Verification items for the finished model (mm, model axes). A direction names the side the tool comes from. Give positions to 0.01 mm unless a question says otherwise; leave off trailing zeros.
from build123d import *

# Parameters (mm, degrees)
SKETCH3_R         = 2.54
CAMERA_LENS_DEPTH = 2.54
SKETCH4_W         = 15.24
SKETCH4_H         = 10.16
CAMERA_BODY_DEPTH = 6.35


with BuildPart() as part:
    # Sketch2 → FOV section 0
    with BuildSketch(Plane(origin=(0, 90.932, 0), x_dir=(1, 0, 0), z_dir=(0, 1, 0))):
        with BuildLine():
            Line((-2.755394972, -1.722121857), (2.755394972, -1.722121857))
            Line((2.755394972, -1.722121857), (2.755394972, 1.722121857))
            Line((2.755394972, 1.722121857), (-2.755394972, 1.722121857))
            Line((-2.755394972, 1.722121857), (-2.755394972, -1.722121857))
        make_face()
    # Sketch1 → FOV section 1
    with BuildSketch(Plane(origin=(0, 0, 0), x_dir=(1, 0, 0), z_dir=(0, 1, 0))):
        with BuildLine():
            Line((-101.6, -63.5), (101.6, -63.5))
            Line((101.6, -63.5), (101.6, 63.5))
            Line((101.6, 63.5), (-101.6, 63.5))
            Line((-101.6, 63.5), (-101.6, -63.5))
        make_face()
    loft()

    # Sketch3 → camera lens (add)
    with BuildSketch(Plane(origin=(0, 90.932, 0), x_dir=(1, 0, 0), z_dir=(0, 1, 0))):
        with Locations(Location((0, 0, 0), (0, 0, 137.312390012))):
            Circle(SKETCH3_R)
    extrude(amount=CAMERA_LENS_DEPTH)

    # Sketch4 → camera body (add)
    with BuildSketch(Plane(origin=(0, 93.472, 0), x_dir=(1, 0, 0), z_dir=(0, 1, 0))):
        Rectangle(SKETCH4_W, SKETCH4_H)
    extrude(amount=CAMERA_BODY_DEPTH)


solid = part.part
(1) Release check for a two-part mould opening along Y. For faces 1 (the flat face through (0, 99.822, 0)), 2 (the cylindrical face through (-2.3, 92.18, -1.08)), 3 (the flat face through (7.62, 97, 0)) record: pulls with the +Y half, pulls with the -Y half, needs draft (parallel to the pull), parting line crosses it, or undercut.
Solved:
face 1: pulls with the +Y half
face 2: undercut
face 3: needs draft
(2) Set-up check for faces 4 (the flat face through (-7.62, 97, 0)), 5 (the flat face through (0, 97, -5.08)), 6 (the flat face through (0, 97, 5.08)): record each of +Z, -Z, +X, -X, +Y, -Y from which the full face is reachable in a straight line by a thin tool's end or side.
Solved:
face 4: +Z, -Z, -X, +Y
face 5: -Z, +X, -X, +Y
face 6: +Z, +X, -X, +Y
(3) Go/stop test with flat-tipped pins: pin 1 (4 mm diameter, centred on y = 20, z = 45, fed in from +X); pin 2 (12 mm diameter, centred on y = 44.5, z = 37.5, fed in from -X); pin 3 (1.9 mm diameter, centred on y = 97, z = 1.5, fed in from -X). Record where each tip stops, or that it passes through.
Solved:
pin 1: stops at x = 82.03
pin 2: stops at x = -59.75
pin 3: stops at x = -7.62
(4) Scan lines: line 1 (Y direction, x = -48, z = -10); line 2 (Y direction, x = 85.5, z = 6); line 3 (X direction, y = 42, z = 8). Record each from-to range of solid material in increasing order.
Solved:
line 1: y = 0 to 49.31
line 2: y = 0 to 14.81
line 3: x = -55.95 to 55.95
